from build123d import *

# Parameters (mm, degrees)
F_10_CLEARANCE_HOLE1_D = 5.1054


with BuildPart() as part:
    # Sketch1 → Revolve1 (revolve)
    with BuildSketch(Plane.XY):
        Polygon((-15.875, 19.05), (-6.604, 19.05), (-6.604, 15.875), (-7.9375, 15.875), (-7.9375, 9.525), (-15.0125, 9.525), (-15.0125, 0), (-20.6375, 0), (-20.6375, 3.1369), (-25.4, 3.1369), (-25.4, 0), (-34.925, 0), (-34.925, 15.875), (-15.875, 15.875), align=None)
    revolve(axis=Axis((0, 0, 0), (0, 1, 0)))

    # #10 Clearance Hole1 (through all)
    with Locations(Plane(origin=(0, 15.875, 0), x_dir=(1, 0, 0), z_dir=(0, 1, 0))):
        with Locations((-21.328108288, 21.328108288), (21.328108288, 21.328108288), (21.328108288, -21.328108288), (-21.328108288, -21.328108288)):
            Hole(F_10_CLEARANCE_HOLE1_D / 2)


solid = part.part
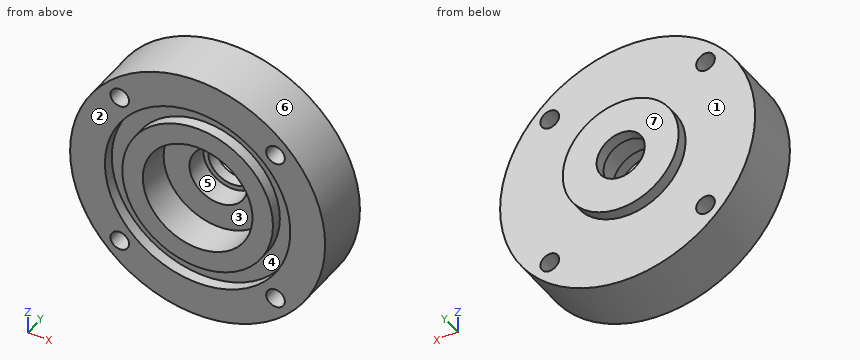
Geometry check sheet. Reference: the model listing, model coordinates, mm. Face numbers are marked on the shaded views. A direction names the side the tool comes from. Round coordinates to 2 decimals unless told otherwise and drop trailing zeros. Order: outer loops, then holes, each group sorted by start corner. A loop starts at its lowest first (then second) coordinate and runs counter-clockwise, first axis right, second up. Notation, with made-up numbers: (86.25, -29.75) -> (102.25, -29.75) arc R30 cw to (102.25, 4.25) -> close; hole circle Ø5 at (47.25, 20). An arc over 180 degrees is marked (long way). Use one line per item in the form item = value.
1. Set-up check for the marked faces 1, 2 and 3: record each of +Z, -Z, +X, -X, +Y, -Y from which the full face is reachable in a straight line by a thin tool's end or side.
Working result:
face_1 = +Y
face_2 = +Z, -Z, +X, -X, -Y
face_3 = -Y
2. Go/stop test with flat-tipped pins: pin 1 (3 mm diameter, centred on x = 19.5, y = 14, fed in from -Z); pin 2 (2 mm diameter, centred on x = -11.5, y = 14.5, fed in from +Z); pin 3 (8 mm diameter, centred on x = -0.5, z = 1, fed in from -Y); pin 4 (4 mm diameter, centred on y = 15, z = -12.5, fed in from +X). Record where each tip stops, or that it passes through.
Working result:
pin_1 = -29.93
pin_2 = 33.31
pin_3 = through
pin_4 = 33.31
3. Mould release check, pull along Z, two halves, no side actions. Record for the marked faces 4, 5, 6 and 7: pulls with the +Z half, pulls with the -Z half, needs draft (parallel to the pull), parting line crosses it, or undercut.
Working result:
face_4 = undercut
face_5 = undercut
face_6 = parting line crosses it
face_7 = needs draft
4. Cross-section at C-C, the plane x = -22. Enter the section's corners in (y, z) (3 decimals).
Working result:
outline = (0, -27.125) -> (15.875, -27.125) -> (15.875, -23.791) -> (0, -23.791) -> close; (0, -18.865) -> (15.875, -18.865) -> (15.875, 18.865) -> (0, 18.865) -> (0, 12.695) -> (3.137, 12.695) -> (3.137, -12.695) -> (0, -12.695) -> close; (0, 23.791) -> (15.875, 23.791) -> (15.875, 27.125) -> (0, 27.125) -> close
5. Scan lines: line 1 along Z through (x, y) = (0, 12.5) (1 decimal); line 2 along Z through (x, y) = (0, 1.1) (1 decimal); line 3 along Z through (x, y) = (-12, 2). Record each from-to range of solid material in increasing order. Write a range as from..to.
Working result:
line_1 = -34.9..-7.9, 7.9..34.9
line_2 = -34.9..-25.4, -20.6..-15, 15..20.6, 25.4..34.9
line_3 = -32.8..-22.39, -16.79..-9.02, 9.02..16.79, 22.39..32.8
